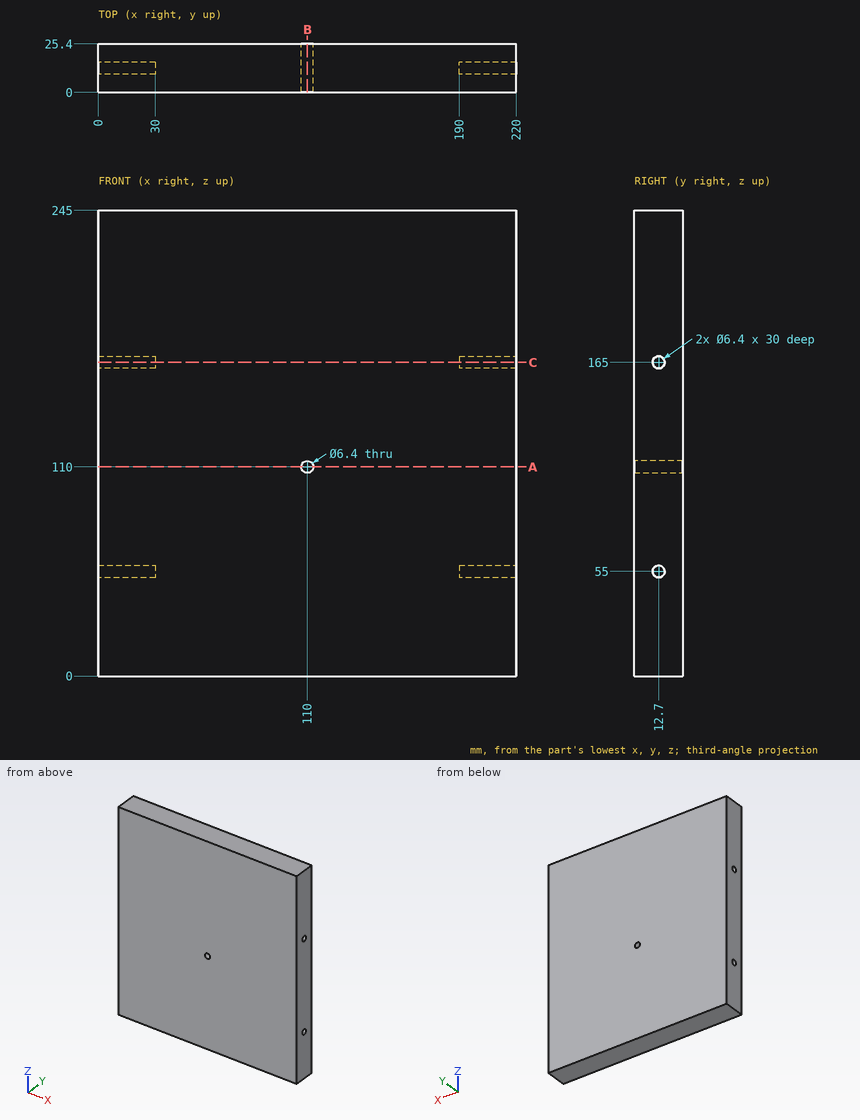
Check sheet for the drawn part. Datum: minimum x, y, z corner. Units: mm. Round coordinates to 2 decimals unless told otherwise and drop trailing zeros. Order: outer loops, then holes, each group sorted by start corner. A loop starts at its lowest first (then second) coordinate and runs counter-clockwise, first axis right, second up.
1. Section check B-B on x = 110. Record the cut outline in (y, z), then the cut area to 3 significant figures.
Final values:
outline: (0, 0) - (25.4, 0) - (25.4, 106.8) - (0, 106.8) - close; (0, 113.2) - (25.4, 113.2) - (25.4, 245) - (0, 245) - close
area: 6,060 mm2
2. Thickness scan on L1, parallel to Z at x = 199.5, y = 12.7; L2, parallel to Y at x = 12, z = 55; L3, parallel to X at y = 15.75, z = 110. Record the ranges inside material, lowest first.
Final values:
L1: z = 0 to 51.8, 58.2 to 161.8, 168.2 to 245
L2: y = 0 to 9.5, 15.9 to 25.4
L3: x = 0 to 106.8, 113.2 to 220
3. Section check A-A on z = 110. Record the cut outline in (x, y).
Final values:
outline: (0, 0) - (106.8, 0) - (106.8, 25.4) - (0, 25.4) - close; (113.2, 0) - (220, 0) - (220, 25.4) - (113.2, 25.4) - close
4. Go/stop test with flat-tipped pins: P1, Ø4, axis at x = 131, y = 15, coming from the -Z side; P2, Ø5, axis at y = 13, z = 55, coming from the -X side; P3, Ø4, axis at y = 12.7, z = 55, coming from the +X side. Record where each tip stops, or that it passes through.
Final values:
P1: stops at z = 0
P2: stops at x = 30
P3: stops at x = 190
5. Section check C-C on z = 165. Record the cut outline in (x, y).
Final values:
outline: (0, 0) - (220, 0) - (220, 9.5) - (190, 9.5) - (190, 15.9) - (220, 15.9) - (220, 25.4) - (0, 25.4) - (0, 15.9) - (30, 15.9) - (30, 9.5) - (0, 9.5) - close
